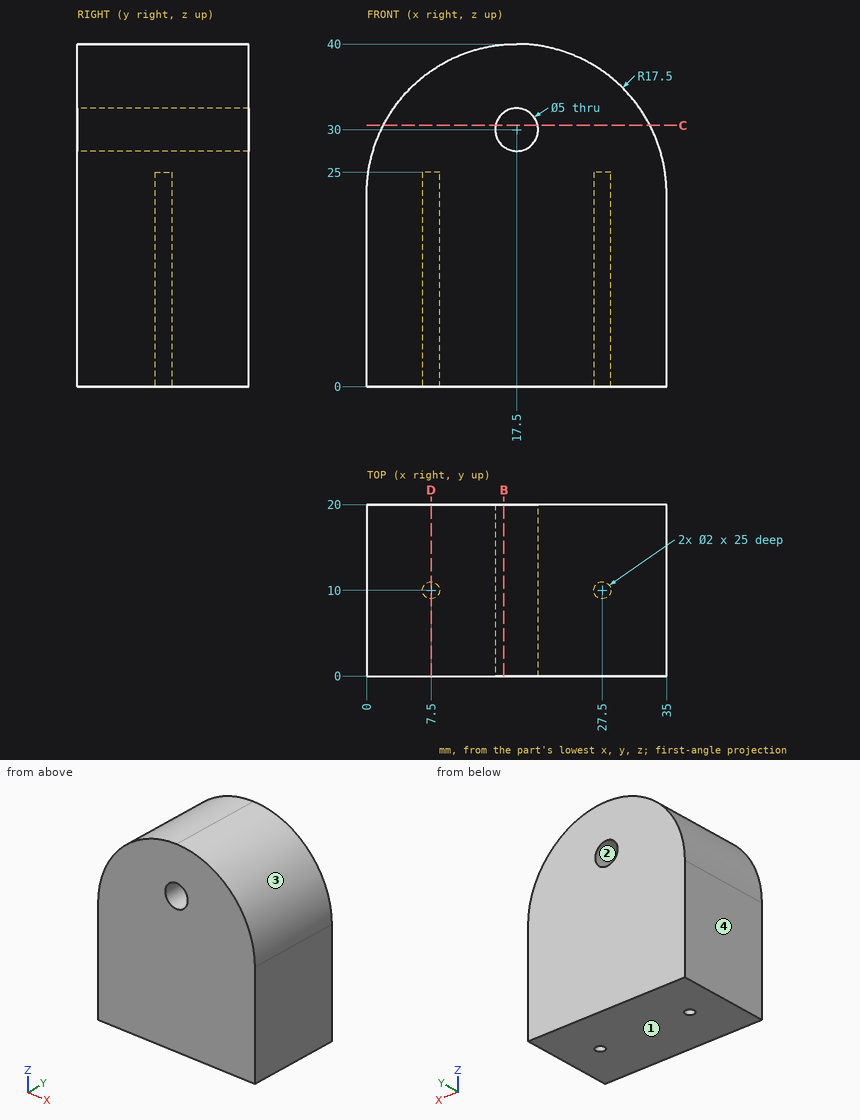
Input: dimensioned drawing with shaded views. Units: mm. Origin: part minimum x, y, z. Coordinates: 2 decimals unless noted, no trailing zeros. Loops run counter-clockwise (first coordinate to the right, second up) from the corner with the lowest first, then second, coordinate; pieces in that order, holes last. Notation, with made-up numbers: M 44.25,50.25 L 66.25,50.25 A32 cw 66.25,82.25 Z; hole C 80,59 d10. An arc over 180 degrees is marked long. One line per item, written item: value. Start each with the question number.
1) Cut plane D-D (x = 7.5). Return loops of the section in (y, z).
2) Cut plane B-B (x = 16). Return loops of the section in (y, z).
3) Draft query along Z for the marked faces 1, 2, 3 and 4. Return one class per face: released by +Z, released by -Z, zero draft, split by the parting line, or undercut.
4) Pin query (flat end, axial travel): P1, Ø1, axis at x = 5.5, y = 10.5, coming from the -Z side; P2, Ø1.8, axis at x = 7.5, y = 10, coming from the -Z side; P3, Ø4.5, axis at x = 17.5, z = 30, coming from the +Y side; P4, Ø1, axis at x = 9.5, y = 11, coming from the +Z side. Return the tip coordinate at first contact, or that it passes through.
5) Cut plane C-C (z = 30.5). Return loops of the section in (x, y), then the cut area to 3 significant figures.
6) Material intervals for L1, parallel to Z at x = 17.5, y = 10.75; L2, parallel to Y at x = 7.5, z = 18; L3, parallel to Z at x = 15.5, y = 11.25, sorted ascending. Write a range as from..to.
Evaluation:
1. outline: M 0,0 L 9,0 L 9,25 L 11,25 L 11,0 L 20,0 L 20,36.86 L 0,36.86 Z
2. outline: M 0,0 L 20,0 L 20,28 L 0,28 Z; M 0,32 L 20,32 L 20,39.94 L 0,39.94 Z
3. face 1: released by -Z
3. face 2: undercut
3. face 3: released by +Z
3. face 4: zero draft
4. P1: z = 0
4. P2: z = 25
4. P3: through
4. P4: z = 38.31
5. outline: M 1.94,0 L 15.05,0 L 15.05,20 L 1.94,20 Z; M 19.95,0 L 33.06,0 L 33.06,20 L 19.95,20 Z
5. area: 525 mm^2
6. L1: 0..27.5, 32.5..40
6. L2: 0..9, 11..20
6. L3: 0..28.5, 31.5..39.89
